Check sheet for the modelled part. Datum: model origin and axes. Units: mm. Round coordinates to 2 decimals unless told otherwise and drop trailing zeros. Order: outer loops, then holes, each group sorted by start corner. A loop starts at its lowest first (then second) coordinate and runs counter-clockwise, first axis right, second up. Notation, with made-up numbers: M 15,55.5 L 61,55.5 A10 ccw 61,62.5 Z; hole C 33,64.25 d3. An arc over 180 degrees is marked long. One line per item, written item: value. Start each with the question number.
(1) Thickness scan on L1, parallel to X at y = 1.5, z = -26.5; L2, parallel to X at y = 6.25, z = 26; L3, parallel to Z at x = 50.5, y = 1.5. Record the ranges inside material, lowest first.
(2) Cross-section at B-B, the plane y = 1.5. Count the separate pieces of the cut face and the enclosed holes in it, and give its area (3 significant figures).
(3) Cross-section at D-D, the plane x = -36. Enter the section's corners in (y, z).
(4) Cross-section at C-C, the plane z = -17.5. Enter the section's corners in (x, y).
(5) Depth check by flat-ended pin: pin 1 Ø2 at (x, y) = (31, 7) entering from +Z; pin 2 Ø3 at (x, y) = (-14.5, 8) entering from +Z; pin 3 Ø6 at (y, z) = (4.5, -36) entering from -X. Enter the tip coordinate at first touch or a pass-through.
(6) Cross-section at A-A, the plane x = 0. Enter the section's corners in (y, z) (3 decimals), and give its area (3 significant figures).
from build123d import *

# Parameters (mm, degrees)
SKETCH_1_R              = 55.25
EXTRUDE_1_DEPTH         = 10
HOLE_WIZARD_3_2_3_2_1_D = 3.2


with BuildPart() as part:
    # 草图1 → 凸台-拉伸1 (new body)
    with BuildSketch(Plane(origin=(0, 0, 0), x_dir=(1, 0, 0), z_dir=(0, 1, 0))):
        Circle(SKETCH_1_R)
    extrude(amount=EXTRUDE_1_DEPTH)

    # Ø3.2 (3.2) 直径孔1 (through all)
    with Locations(Plane(origin=(0, 10, -52.525), x_dir=(0, 0, 1), z_dir=(0, 1, 0))):
        with Locations((0, 0), (26.2625, -45.487984334), (78.7875, -45.487984334), (105.05, 0), (78.7875, 45.487984334), (26.2625, 45.487984334)):
            Hole(HOLE_WIZARD_3_2_3_2_1_D / 2)


solid = part.part
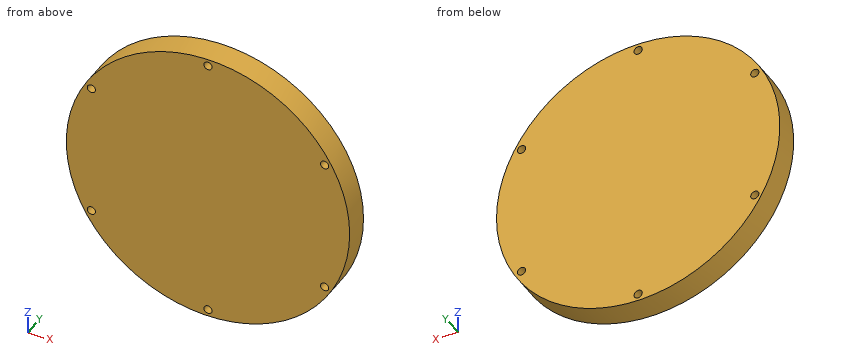
Values found:
1. L1: -48.48 to -47.07, -43.91 to 43.91, 47.07 to 48.48
1. L2: -48.75 to -47.07, -43.91 to 43.91, 47.07 to 48.75
1. L3: -22.41 to 22.41
2. separate pieces: 1
2. enclosed holes: 6
2. area: 9,540 mm^2
3. outline: M 0,-41.91 L 10,-41.91 L 10,41.91 L 0,41.91 Z
4. outline: M -52.41,0 L 52.41,0 L 52.41,10 L -52.41,10 Z
5. pin 1: z = 46.4
5. pin 2: z = 53.7
5. pin 3: x = -44.31
6. outline: M 0,-55.25 L 10,-55.25 L 10,-54.125 L 0,-54.125 Z; M 0,-50.925 L 10,-50.925 L 10,50.925 L 0,50.925 Z; M 0,54.125 L 10,54.125 L 10,55.25 L 0,55.25 Z
6. area: 1,040 mm^2
